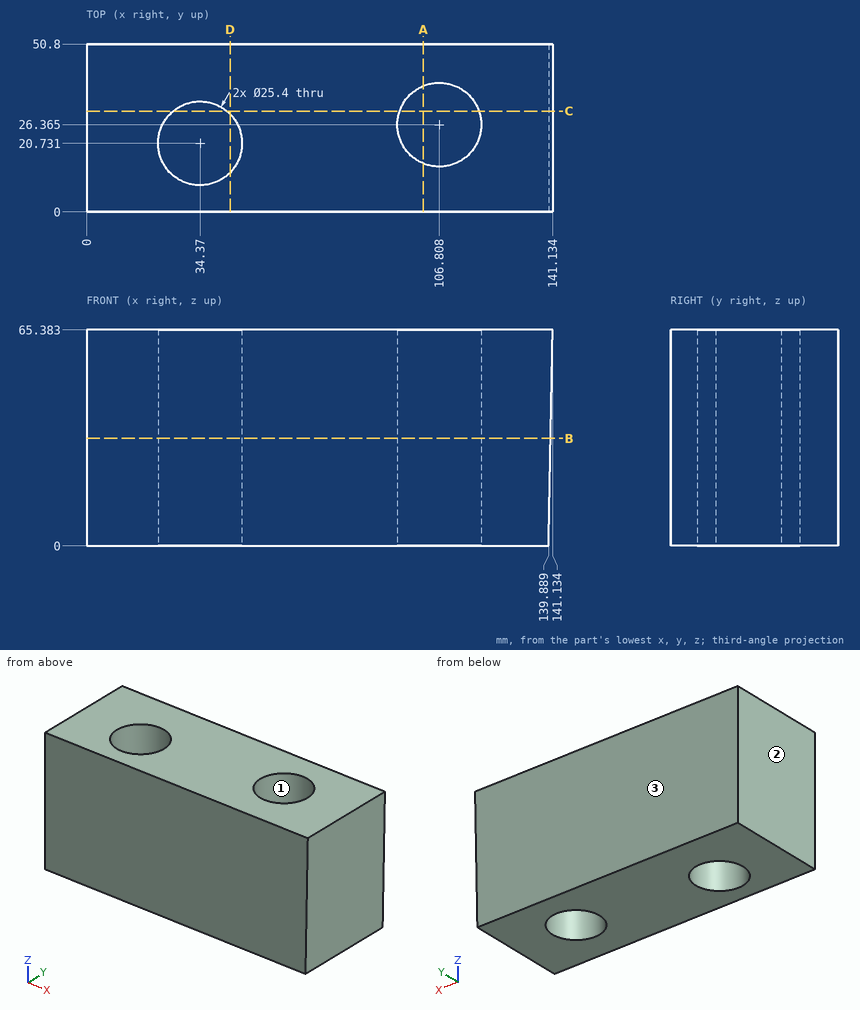
Could you check a few things on this drawing? It's one solid part, dimensions in mm from its lowest x, y, z. Coordinates: 2 decimals unless noted, no trailing zeros. Write each loop counter-clockwise with the first axis right and the second up, starting at its lowest first coordinate (ties: lowest second). Pieces come first, ordered by that corner, then holes. Notation, with made-up numbers: (-13.5, -16) - (0.5, -16) arc R23 ccw to (0.5, -3) - close; hole circle Ø7 at (75, -18.5). An arc over 180 degrees is marked (long way). Put each result on its own line as item: value. Start each with the question number.
Q1. I want a section at C-C on y = 30.5. Write out the boundary of the cut face in (x, z) (1 decimal), plus the area to 3 significant figures.
Q2. I want a section at A-A on x = 102. Write out the boundary of the cut face in (y, z), plus the area to 3 significant figures.
Q3. I'm going to push flat-ended pins straight in: P1, Ø8, axis at y = 45, z = 53.5, coming from the +X side; P2, Ø20.5, axis at x = 106.81, y = 26.36, coming from the +Z side; P3, Ø2, axis at y = 38.5, z = 23.5, coming from the +X side (1 decimal). Where does each tip first touch, or does it pass through?
Q4. I want a section at D-D on x = 43.5. Write out the boundary of the cut face in (y, z), plus the area to 3 significant figures.
Q5. I want a section at B-B on z = 32.5. Write out the boundary of the cut face in (x, y) (1 decimal), plus the area to 3 significant figures.
Q6. Thinking about a two-plate mould opening in Y: for the marked faces 1, 2 and 3, which applies, pulls with the +Y half, pulls with the -Y half, needs draft (parallel to the pull), parting line crosses it, or undercut?
Q7. Please list where these lines run through material, in increasing order: L1, parallel to X at y = 27.5, z = 52.5 (1 decimal); L2, parallel to X at y = 31.5, z = 31.5 (1 decimal); L3, parallel to X at y = 34, z = 36 (1 decimal).
Checks:
1. outline: (0, 0) - (26.3, 0) - (26.3, 65.4) - (0, 65.4) - close; (42.5, 0) - (94.8, 0) - (94.8, 65.4) - (42.5, 65.4) - close; (118.8, 0) - (139.9, 0) - (141.1, 65.4) - (118.8, 65.4) - close
1. area: 6,560 mm²
2. outline: (0, 0) - (14.61, 0) - (14.61, 65.38) - (0, 65.38) - close; (38.12, 0) - (50.8, 0) - (50.8, 65.38) - (38.12, 65.38) - close
2. area: 1,780 mm²
3. P1: x = 140.98
3. P2: through
3. P3: x = 140.4
4. outline: (0, 0) - (11.9, 0) - (11.9, 65.38) - (0, 65.38) - close; (29.56, 0) - (50.8, 0) - (50.8, 65.38) - (29.56, 65.38) - close
4. area: 2,170 mm²
5. outline: (0, 0) - (140.5, 0) - (140.5, 50.8) - (0, 50.8) - close; hole circle Ø25.4 at (34.4, 20.7); hole circle Ø25.4 at (106.8, 26.4)
5. area: 6,120 mm²
6. face 1: undercut
6. face 2: needs draft
6. face 3: pulls with the +Y half
7. L1: 0 to 23.6, 45.1 to 94.2, 119.5 to 140.9
7. L2: 0 to 27.6, 41.1 to 95.2, 118.4 to 140.5
7. L3: 0 to 96.7, 117 to 140.6
